```python
from build123d import *

# Parameters (mm, degrees)
F0_R     = 101.6
F1_DEPTH = 76.2
F3_D     = 152.4
F4_R     = 5.08


with BuildPart() as f1:
    # F0 (on Front) → F1 (new body)
    with BuildSketch(Plane.XZ):
        Circle(F0_R)
    extrude(amount=F1_DEPTH)

    # F3 (through all)
    with Locations(Plane.XZ.offset(76.2)):
        with Locations((0, 0)):
            Hole(F3_D / 2)

    # F4
    f4_edges = [f1.edges().sort_by_distance(p)[0] for p in [
        (-101.6, -76.2, 0),
        (-101.6, 0, 0),
        (-76.2, 0, 0),
        (-76.2, -76.2, 0),
    ]]
    fillet(f4_edges, radius=F4_R)


solid = f1.part
```
Geometry check sheet. Reference: the model listing, model coordinates, mm. Coordinates: 2 decimals unless noted, no trailing zeros. Order: outer loops, then holes, each group sorted by start corner. A loop starts at its lowest first (then second) coordinate and runs counter-clockwise, first axis right, second up. Notation, with made-up numbers: (88.5, -23.75) - (122.5, -23.75) arc R21 ccw to (122.5, 14.25) - close; hole circle Ø10 at (-4, -16). An arc over 180 degrees is marked (long way). Answer as a JSON object with one key per item and string values. Group by question number.
Item 1: Draft check along Z on faces 1 (the face through (-50.5, -76.2, -63.9)), 2 (the face through (-22.025, -37.638, -99.184)), 3 (the face through (60.47, -37.638, -46.367)). Enter one of: +Z half, -Z half, draft (parallel to the pull), parting line (faces both ways), or undercut.
Item 2: Scan lines: probe 1 along Z at (x, y) = (0, -31); probe 2 along X at (y, z) = (-72, 41); probe 3 along Z at (x, y) = (60.5, -8). Record each from-to range of solid material in increasing order.
Item 3: Sectioned sample at A-A, the plane z = 0. Record the cut outline in (x, y).
Item 4: Sectioned sample at B-B, the plane x = 0. Record the cut outline in (y, z), and give its area (3 significant figures).
Item 5: Depth check by flat-ended pin: pin 1 Ø3 at (y, z) = (-65.5, -29) entering from +X; pin 2 Ø6 at (y, z) = (-8.5, 6) entering from +X; pin 3 Ø12 at (x, y) = (54.5, -33) entering from +Z. Enter the tip coordinate at first touch or a pass-through.
Item 6: Sectioned sample at C-C, the plane y = -50. Record the cut outline in (x, z).
Resolved:
{
 "1": {"face 1": "draft", "face 2": "parting line", "face 3": "undercut"},
 "2": {"probe 1": "-101.6 to -76.2, 76.2 to 101.6", "probe 2": "-92.88 to -64.32, 64.32 to 92.88", "probe 3": "-81.62 to -46.33, 46.33 to 81.62"},
 "3": {"outline": "(-101.6, -71.12) arc R5.08 ccw to (-96.52, -76.2) - (-81.28, -76.2) arc R5.08 ccw to (-76.2, -71.12) - (-76.2, -5.08) arc R5.08 ccw to (-81.28, 0) - (-96.52, 0) arc R5.08 ccw to (-101.6, -5.08) - close; (76.2, -71.12) arc R5.08 ccw to (81.28, -76.2) - (96.52, -76.2) arc R5.08 ccw to (101.6, -71.12) - (101.6, -5.08) arc R5.08 ccw to (96.52, 0) - (81.28, 0) arc R5.08 ccw to (76.2, -5.08) - close"},
 "4": {"outline": "(-76.2, -96.52) arc R5.08 ccw to (-71.12, -101.6) - (-5.08, -101.6) arc R5.08 ccw to (0, -96.52) - (0, -81.28) arc R5.08 ccw to (-5.08, -76.2) - (-71.12, -76.2) arc R5.08 ccw to (-76.2, -81.28) - close; (-76.2, 81.28) arc R5.08 ccw to (-71.12, 76.2) - (-5.08, 76.2) arc R5.08 ccw to (0, 81.28) - (0, 96.52) arc R5.08 ccw to (-5.08, 101.6) - (-71.12, 101.6) arc R5.08 ccw to (-76.2, 96.52) - close", "area": "3,830 mm^2"},
 "5": {"pin 1": "x = 97.81", "pin 2": "x = 101.56", "pin 3": "z = 89.28"},
 "6": {"outline": "circle Ø203.2 at (0, 0); hole circle Ø152.4 at (0, 0)"}
}
